Work out the finished part from the listing and answer in its coordinate system (mm). Give positions to 0.01 mm unless a question says otherwise; leave off trailing zeros. Write each loop counter-clockwise with the first axis right and the second up, starting at its lowest first coordinate (ties: lowest second). Pieces come first, ordered by that corner, then holes. Notation, with made-up numbers: (79.25, -39) - (99.25, -39) arc R27 ccw to (99.25, -3) - close; hole circle Ø9 at (58.5, -11.75). An arc over 180 degrees is marked (long way). Write item = value, one per line.
Autodesk Inventor part; units mm, degrees
ref_plane "YZ Plane" through (0, 0, 0) normal (1, 0, 0) x (0, 1, 0)
ref_plane "XZ Plane" through (0, 0, 0) normal (0, 1, 0) x (-1, 0, 0)
ref_plane "XY Plane" through (0, 0, 0) normal (0, 0, 1) x (1, 0, 0)
sketch "Sketch1" plane through (0, 0, 0) normal (0, 1, 0) x (-1, 0, 0)
  arc A0 (45.4572, -61.1563) -> (62.9817, -42.8923) centre (54.9831, -52.757) ccw
  circle A1 centre (54.9831, -52.757) radius 3.75
  circle A2 centre (73.1804, 21.2382) radius 3.75 construction
  circle A3 centre (18.1974, 73.9952) radius 3.75 construction
  circle A4 centre (-54.9831, 52.757) radius 3.75 construction
  circle A5 centre (-73.1804, -21.2382) radius 3.75 construction
  circle A6 centre (-18.1974, -73.9952) radius 3.75 construction
  arc A7 (62.9817, -42.8923) -> (72.047, 24.8128) centre (0, 0) ccw
  arc A8 (-66.4803, 37.2399) -> (-72.047, -24.8128) centre (0, 0) ccw
  arc A9 (-20.846, -73.2932) -> (4.312, -76.0779) centre (-8.3834, -75.7374) ccw
  arc A10 (-70.8376, -28.0798) -> (-57.7316, -49.7343) centre (-65.19, -39.455) ccw
  arc A11 (-50.6143, 56.9617) -> (-66.4803, 37.2399) centre (-59.3719, 47.7642) ccw
  arc A12 (14.3787, 74.8311) -> (-10.9263, 75.4126) centre (1.7505, 76.1799) ccw
  arc A13 (68.1207, 34.1469) -> (53.1773, 54.5767) centre (61.5032, 44.9866) ccw
  circle A14 centre (-8.3834, -75.7374) radius 3.75
  circle A15 centre (-65.19, -39.455) radius 3.75
  circle A16 centre (-59.3719, 47.7642) radius 3.75
  circle A17 centre (1.7505, 76.1799) radius 3.75
  circle A18 centre (61.5032, 44.9866) radius 3.75
  arc A19 (-14.535, -74.8009) -> (-12.0993, -75.2333) centre (0, 0) ccw
  arc A20 (4.312, -76.0779) -> (45.4572, -61.1563) centre (0, 0) ccw
  arc A21 (-72.047, -24.8128) -> (-70.8376, -28.0798) centre (0, 0) ccw
  arc A22 (-57.7316, -49.7343) -> (-20.846, -73.2932) centre (0, 0) ccw
  arc A23 (14.535, 74.8009) -> (14.3787, 74.8311) centre (0, 0) ccw
  arc A24 (-10.9263, 75.4126) -> (-50.6143, 56.9617) centre (0, 0) ccw
  arc A25 (72.047, 24.8128) -> (68.1207, 34.1469) centre (0, 0) ccw
  arc A26 (53.1773, 54.5767) -> (14.535, 74.8009) centre (0, 0) ccw
  point P0 (73.9952, -18.1974)
  dimension "d7" = 25.4
  dimension "d15" = 7.5
  dimension "d18" = 360
  dimension "d22" = 52.5
  dimension "d23" = 80
  dimension "d24" = 52.5
  dimension "d25" = 52.5
  dimension "d26" = 52.5
  dimension "d27" = 70
extrude "Extrusion1" add sketch "Sketch1" along normal blind 1.905
properties part number "Base_bottom"
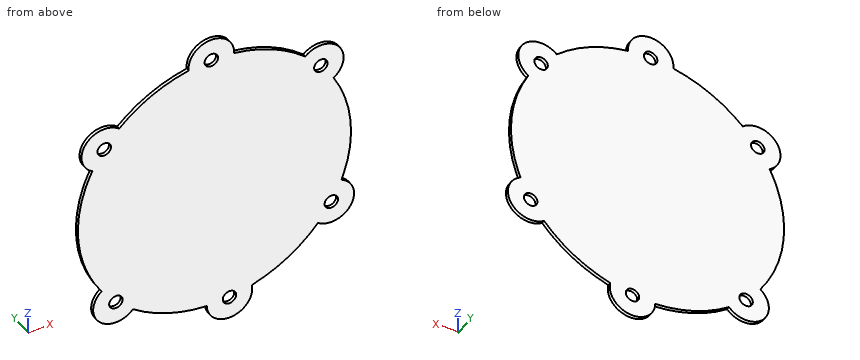
1. Given pin 1 (7 mm diameter, centred on x = -54.98, z = -52.76, fed in from -Y), flat-ended and moving along its own axis, determine where the tip first touches the part or whether it passes through.
Solution:
pin_1 = through
2. Straight lines are drawn through the part: line 1 (X direction, y = 1.45, z = -50); line 2 (Z direction, x = 69.5, y = 0.95); line 3 (Z direction, x = -53.5, y = 1.6). For each, find the intervals that lie inside material, in ascending order.
Solution:
line_1 = -67.38 to -57.53, -52.44 to 57.5, 58.11 to 72.27
line_2 = -51.4 to 31.24, 40.1 to 55.43
line_3 = -65.37 to -56.2, -49.31 to 54.85
3. Find section C-C, the plane x = 17.5. Give the vertices of the cut face in (y, z) (3 decimals).
Solution:
outline = (0, -84.579) - (1.905, -84.579) - (1.905, 74.163) - (0, 74.163) - close
4. Find section A-A, the plane y = 1.15. Give the number of separate pieces and of enclosed holes in the cut face, then the cut area to 3 significant figures.
Solution:
separate_pieces = 1
enclosed_holes = 6
area = 19,600 mm^2
5. Find section B-B, the plane z = 31.5. Give the vertices of the cut face in (x, y) (3 decimals).
Solution:
outline = (-69.384, 0) - (69.384, 0) - (69.384, 1.905) - (-69.384, 1.905) - close
